Source: CAD feature listing. Evaluate the final solid. Frame: model axes, mm. Face numbers are marked on the shaded views. Round coordinates to 2 decimals unless told otherwise and drop trailing zeros. Order: outer loops, then holes, each group sorted by start corner. A loop starts at its lowest first (then second) coordinate and runs counter-clockwise, first axis right, second up. Notation, with made-up numbers: (31, 47) -> (45, 47) arc R17 ccw to (45, 68) -> close; hole circle Ø6 at (67.25, 67). An arc over 180 degrees is marked (long way). One line per item, written item: value. Start each with the question number.
1) Section A-A (y = 7). Return the cut outline in (x, z).
2) Mould query, pull axis Y, two halves, no side actions, for the marked faces 1 and 2. Classes: pulls with the +Y half, pulls with the -Y half, needs draft (parallel to the pull), parting line crosses it, or undercut.
3) Pin query (flat end, axial travel): P1, Ø13.5, axis at x = 9.5, y = 10, coming from the +Z side. Return the tip coordinate at first contact, or that it passes through.
4) Ray query, L1, parallel to X at y = -39.5, z = 0.7; L2, parallel to Y at x = 15, z = 0.9; L3, parallel to Z at x = -0.5, y = -26.5. Return the intervals inside material, ascending.
5) Section B-B (z = 1.4). State how many separate pieces and enclosed holes the cut face has, and give its area (3 significant figures).
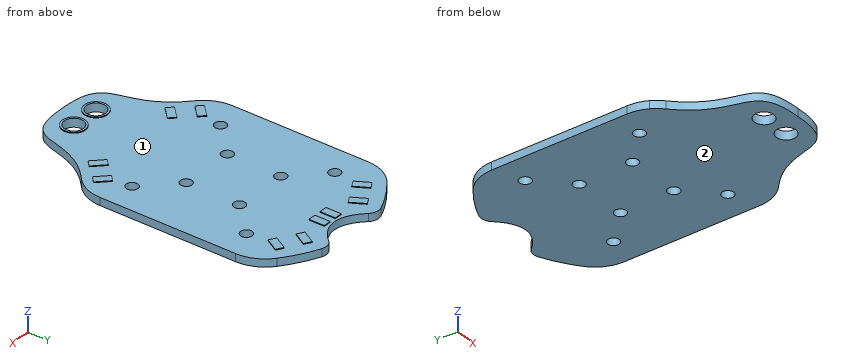
```python
from build123d import *

# Parameters (mm, degrees)
F0_R     = 2.5
F0_R_2   = 1.5
F1_DEPTH = 2
F2_W     = 2
F2_H     = 4
F2_R     = 3
F2_R_2   = 2.5
F3_DEPTH = 0.2


with BuildPart() as f1:
    # F0 (on Top) → F1 (new body)
    with BuildSketch(Plane.XY):
        with BuildLine():
            Line((22.5, -17.5992111466), (22.5, 17.9769920821))
            ThreePointArc((22.5, 17.9769920821), (21.4916275861, 22.3531357443), (18.6698733295, 25.8467228969))
            add(Edge.make_bspline(
                [(10.0202101022, 30.9724353404), (12.9351645554, 29.7852274215), (15.8255721427, 28.076656607), (18.6698733295, 25.8467228969)],
                knots=[32.3872433875, 32.3872433875, 32.3872433875, 32.3872433875, 41.0712182165, 41.0712182165, 41.0712182165, 41.0712182165], degree=3))
            ThreePointArc((10.0202101022, 30.9724353404), (8.4843597996, 31.1666740134), (7.0561575797, 30.569343926))
            add(Edge.make_bspline(
                [(-6.6778963244, 30.2220172158), (-2.1223269725, 25.2559450952), (2.9587594632, 25.5243336352), (7.0561575797, 30.569343926)],
                knots=[1.2111660498, 1.2111660498, 1.2111660498, 1.2111660498, 14.8998546864, 14.8998546864, 14.8998546864, 14.8998546864], degree=3))
            ThreePointArc((-6.6778963244, 30.2220172158), (-8.2314180106, 31.1211658606), (-10.0202101022, 30.9724353404))
            add(Edge.make_bspline(
                [(-18.6698733295, 25.8467228969), (-15.8255721427, 28.076656607), (-12.9351645554, 29.7852274215), (-10.0202101022, 30.9724353404)],
                knots=[3.9287817835, 3.9287817835, 3.9287817835, 3.9287817835, 12.6127566125, 12.6127566125, 12.6127566125, 12.6127566125], degree=3))
            ThreePointArc((-18.6698733295, 25.8467228969), (-21.4916275861, 22.3531357443), (-22.5, 17.9769920821))
            Line((-22.5, 17.9769920821), (-22.5, -17.5992111466))
            ThreePointArc((-22.5, -17.5992111466), (-22.1738774189, -20.1322124661), (-21.216780863, -22.5))
            ThreePointArc((-21.216780863, -22.5), (-20.2661626921, -23.8989505888), (-19.0933749805, -25.1176821592))
            add(Edge.make_bspline(
                [(-19.0933749805, -25.1176821592), (-6.7235541682, -35.9654817875), (-16.745618261, -45.2509330365), (0, -45)],
                knots=[2.3473845635, 2.3473845635, 2.3473845635, 2.3473845635, 31.8198051534, 31.8198051534, 31.8198051534, 31.8198051534], degree=3))
            add(Edge.make_bspline(
                [(19.0933749805, -25.1176821592), (6.7235541682, -35.9654817875), (16.745618261, -45.2509330365), (0, -45)],
                knots=[2.3473845635, 2.3473845635, 2.3473845635, 2.3473845635, 31.8198051534, 31.8198051534, 31.8198051534, 31.8198051534], degree=3))
            ThreePointArc((19.0933749805, -25.1176821592), (21.6086154218, -21.7263318254), (22.5, -17.5992111466))
        make_face()
        with Locations((-3.75, -39)):
            Circle(F0_R, mode=Mode.SUBTRACT)
        with Locations((-15, -15)):
            Circle(F0_R_2, mode=Mode.SUBTRACT)
        with Locations((-7, -7)):
            Circle(F0_R_2, mode=Mode.SUBTRACT)
        with Locations((3.75, -39)):
            Circle(F0_R, mode=Mode.SUBTRACT)
        with Locations((7, -7)):
            Circle(F0_R_2, mode=Mode.SUBTRACT)
        with Locations((15, -15)):
            Circle(F0_R_2, mode=Mode.SUBTRACT)
        with Locations((-7, 7)):
            Circle(F0_R_2, mode=Mode.SUBTRACT)
        with Locations((-15, 15)):
            Circle(F0_R_2, mode=Mode.SUBTRACT)
        with Locations((7, 7)):
            Circle(F0_R_2, mode=Mode.SUBTRACT)
        with Locations((15, 15)):
            Circle(F0_R_2, mode=Mode.SUBTRACT)
    extrude(amount=F1_DEPTH)

    # F2 (on face) → F3 (join)
    with BuildSketch(Plane.XY.offset(2)):
        Polygon((-16.4196526402, 23.6817868025), (-14.4196526402, 20.2176851873), (-12.6876018326, 21.2176851873), (-14.6876018326, 24.6817868025), align=None)
        Polygon((-11.0663396811, 26.9043505312), (-9.0663396811, 23.4402489161), (-7.3342888736, 24.4402489161), (-9.3342888736, 27.9043505312), align=None)
        with Locations((-1.8889066383, 24.0563029559)):
            Rectangle(F2_W, F2_H)
        with Locations((1.8889066383, 24.0563029559)):
            Rectangle(F2_W, F2_H)
        Polygon((9.3342888736, 27.9043505312), (7.3342888736, 24.4402489161), (9.0663396811, 23.4402489161), (11.0663396811, 26.9043505312), align=None)
        Polygon((12.6876018326, 21.2176851873), (14.4196526402, 20.2176851873), (16.4196526402, 23.6817868025), (14.6876018326, 24.6817868025), align=None)
        Polygon((-17.3788340109, -23.5849192398), (-14.5510007349, -20.755898391), (-15.9655111593, -19.341981753), (-18.7933444353, -22.1710026018), align=None)
        Polygon((-14.4555578038, -26.6683889275), (-13.0410473794, -28.0823055655), (-10.2132141034, -25.2532847167), (-11.6277245278, -23.8393680786), align=None)
        Polygon((10.2132141034, -25.2532847167), (13.0410473794, -28.0823055655), (14.4555578038, -26.6683889275), (11.6277245278, -23.8393680786), align=None)
        Polygon((14.5510007349, -20.755898391), (17.3788340109, -23.5849192398), (18.7933444353, -22.1710026018), (15.9655111593, -19.341981753), align=None)
        with Locations((-3.75, -39)):
            Circle(F2_R)
        with Locations((-3.75, -39)):
            Circle(F2_R_2, mode=Mode.SUBTRACT)
        with Locations((3.75, -39)):
            Circle(F2_R)
        with Locations((3.75, -39)):
            Circle(F2_R_2, mode=Mode.SUBTRACT)
    extrude(amount=F3_DEPTH)


solid = f1.part
```
Findings:
1. outline: (-22.5, 0) -> (-8.5, 0) -> (-8.5, 2) -> (-22.5, 2) -> close; (-5.5, 0) -> (5.5, 0) -> (5.5, 2) -> (-5.5, 2) -> close; (8.5, 0) -> (22.5, 0) -> (22.5, 2) -> (8.5, 2) -> close
2. face 1: undercut
2. face 2: needs draft
3. P1: z = 2
4. L1: -11.1 to -6.2, -1.3 to 1.3, 6.2 to 11.1
4. L2: -29.68 to -16.5, -13.5 to 13.5, 16.5 to 28.42
4. L3: 0 to 2
5. separate pieces: 1
5. enclosed holes: 10
5. area: 2,780 mm2
